The listing builds one solid part. Answer for the finished solid, in the listing's coordinates (mm). A direction names the side the tool comes from. Give positions to 0.01 mm unless a question says otherwise; leave off trailing zeros. Write each loop counter-clockwise with the first axis right and the second up, starting at its lowest first coordinate (ties: lowest second). Pieces come first, ordered by that corner, then holes. Notation, with made-up numbers: M 18,37.25 L 50,37.25 A16 cw 50,67.25 Z; hole C -27.75,-29.75 d10. An arc over 180 degrees is marked long. Return JSON: item names as keys, results as strings.
from build123d import *

# Parameters (mm, degrees)
F1_DEPTH = 28.575
F3_DEPTH = 44.45
F4_R     = 12.7
F5_DEPTH = 57.15
F6_R     = 5.08
F7_DEPTH = 25.4


with BuildPart() as f1:
    # F0 (on Front) → F1 (new body, symmetric)
    with BuildSketch(Plane.XZ):
        Polygon((31.75, 12.7), (31.75, 0), (95.25, 0), (95.25, 12.7), (76.2, 12.7), (76.2, 21.59), (127, 21.59), (127, 88.9), (0, 88.9), (0, 21.59), (50.8, 21.59), (50.8, 12.7), align=None)
    extrude(amount=F1_DEPTH, both=True)

    # F2 (on face) → F3 (cut)
    with BuildSketch(Plane.XZ.offset(28.575)):
        with BuildLine():
            Line((0, 88.9), (0, 34.29))
            Line((0, 34.29), (16.044335, 34.29))
            Line((16.044335, 34.29), (44.050399, 79.836248))
            ThreePointArc((44.050399, 79.836248), (52.771084, 86.522822), (63.5, 88.9))
            Line((63.5, 88.9), (0, 88.9))
        make_face()
        with BuildLine():
            Line((127, 88.9), (63.5, 88.9))
            ThreePointArc((63.5, 88.9), (74.228916, 86.522822), (82.949601, 79.836248))
            Line((82.949601, 79.836248), (111.294335, 34.29))
            Line((111.294335, 34.29), (127, 34.29))
            Line((127, 34.29), (127, 88.9))
        make_face()
    extrude(amount=-F3_DEPTH, mode=Mode.SUBTRACT)

    # F4 (on face) → F5 (cut)
    with BuildSketch(Plane.XZ.offset(28.575)):
        with Locations((63.5, 63.5)):
            Circle(F4_R)
    extrude(amount=-F5_DEPTH, mode=Mode.SUBTRACT)

    # F6 (on face) → F7 (cut)
    with BuildSketch(Plane.XY.offset(88.9)):
        with Locations((63.5, -6.35)):
            Circle(F6_R)
    extrude(amount=-F7_DEPTH, mode=Mode.SUBTRACT)


solid = f1.part
Item 1: Which of the six approach directions +Z, -Z, +X, -X, +Y, -Y give full straight-line access (tool end or side, diameter ignored) to faces 4 (the flat face through (29.85, -6.66, 56.74)), 5 (the flat face through (25, 0, 21.59)), 6 (the flat face through (109, 15.875, 68))?
Geometry results:
{"face 4": "+Z, -X, -Y", "face 5": "-X, +Y, -Y", "face 6": "+Z, +X, -Y"}
Item 2: A cutting plane is placed at C-C, the plane x = 10.5. Write down the section's boundary in (y, z) (3 decimals).
Geometry results:
{"outline": "M -28.575,21.59 L 28.575,21.59 L 28.575,88.9 L 15.875,88.9 L 15.875,34.29 L -28.575,34.29 Z"}
Item 3: Determine the mould class of faces 1 (the flat face through (96.924, -6.661, 57.382)), 2 (the cylindrical face through (68.345, -4.824, 82.116)), 3 (the flat face through (63, 28.575, 45)) for opening direction X: +X half, -X half, draft (parallel to the pull), parting line (faces both ways), or undercut.
Geometry results:
{"face 1": "+X half", "face 2": "undercut", "face 3": "draft"}
Item 4: Find the intervals of material crossed by line 1 (Z direction, x = 93, y = 25.5); line 2 (Z direction, x = 63.5, y = 15); line 3 (Z direction, x = 14, y = -22), in increasing order.
Geometry results:
{"line 1": "z = 0 to 12.7, 21.59 to 88.9", "line 2": "z = 0 to 50.8, 76.2 to 88.9", "line 3": "z = 21.59 to 34.29"}
Item 5: A cutting plane is placed at D-D, the plane y = 24. Write down the section's boundary in (x, z).
Geometry results:
{"outline": "M 0,21.59 L 50.8,21.59 L 50.8,12.7 L 31.75,12.7 L 31.75,0 L 95.25,0 L 95.25,12.7 L 76.2,12.7 L 76.2,21.59 L 127,21.59 L 127,88.9 L 0,88.9 Z; hole C 63.5,63.5 d25.4"}
Item 6: A cutting plane is placed at B-B, the plane z = 63.5. Write down the section's boundary in (x, y) (3 decimals), plus the area to 3 significant figures.
Geometry results:
{"outline": "M 0,15.875 L 34.005,15.875 L 34.005,-28.575 L 50.8,-28.575 L 50.8,28.575 L 0,28.575 Z; M 76.2,-28.575 L 93.116,-28.575 L 93.116,15.875 L 127,15.875 L 127,28.575 L 76.2,28.575 Z", "area": "2,790 mm2"}
Item 7: A cutting plane is placed at A-A, the plane y = 8. Write down the section's boundary in (x, z), plus the area to 3 significant figures.
Geometry results:
{"outline": "M 0,21.59 L 50.8,21.59 L 50.8,12.7 L 31.75,12.7 L 31.75,0 L 95.25,0 L 95.25,12.7 L 76.2,12.7 L 76.2,21.59 L 127,21.59 L 127,34.29 L 111.29,34.29 L 82.95,79.84 A25.4 ccw 63.5,88.9 A25.4 ccw 44.05,79.84 L 16.04,34.29 L 0,34.29 Z; hole C 63.5,63.5 d25.4", "area": "5,440 mm2"}
Item 8: Given pin 1 Ø2 at (x, y) = (54, -20) entering from -Z; pin 2 Ø10 at (y, z) = (5.5, 6.5) entering from +X; pin 3 Ø13 at (x, y) = (5.5, -12.5) entering from +Z; pin 4 Ø4 at (y, z) = (-2, 4) entering from -X, each flat-ended and moving along its own axis, determine where each tip first touches the part or whether it passes through.
Geometry results:
{"pin 1": "stops at z = 0", "pin 2": "stops at x = 95.25", "pin 3": "stops at z = 34.29", "pin 4": "stops at x = 31.75"}
